```python
from build123d import *

# Parameters (mm, degrees)
SKETCH1_R                  = 31
BOSS_EXTRUDE1_DEPTH        = 4
F_3_2_3_2_DIAMETER_HOLE1_D = 3.2
F_3_0_3_DIAMETER_HOLE1_D   = 3
SKETCH6_W                  = 4
SKETCH6_H                  = 4
CUT_EXTRUDE2_DEPTH         = 45.022721406


with BuildPart() as part:
    # Sketch1 → Boss-Extrude1 (new body)
    with BuildSketch(Plane(origin=(0, 0, 0), x_dir=(1, 0, 0), z_dir=(0, 1, 0))):
        with Locations(Location((0, 0, 0), (0, 0, 270))):
            Circle(SKETCH1_R)
    extrude(amount=BOSS_EXTRUDE1_DEPTH)

    # Ø3.2 (3.2) Diameter Hole1 (through all)
    with Locations(Plane(origin=(0, 4, 0), x_dir=(1, 0, 0), z_dir=(0, 1, 0))):
        with Locations((-27.5, 0), (27.5, 0), (0, 27.5), (0, -27.5)):
            Hole(F_3_2_3_2_DIAMETER_HOLE1_D / 2)

    # Ø3.0 (3) Diameter Hole1 (through all)
    with Locations(Plane(origin=(0, 4, 0), x_dir=(1, 0, 0), z_dir=(0, 1, 0))):
        with Locations((-16.135, 0)):
            Hole(F_3_0_3_DIAMETER_HOLE1_D / 2)

    # Sketch6 → Cut-Extrude2 (cut, through all)
    with BuildSketch(Plane(origin=(0, 4, 0), x_dir=(1, 0, 0), z_dir=(0, 1, 0))):
        with Locations((0, 16.135)):
            Rectangle(SKETCH6_W, SKETCH6_H)
    extrude(amount=-CUT_EXTRUDE2_DEPTH, mode=Mode.SUBTRACT)


solid = part.part
```
Geometry: final body of the model. Coordinates: model frame, mm. A direction names the side the tool comes from. Coordinates: 2 decimals unless noted, no trailing zeros. Loops run counter-clockwise (first coordinate to the right, second up) from the corner with the lowest first, then second, coordinate; pieces in that order, holes last. Notation, with made-up numbers: M -21,41.25 L 5,41.25 A23 cw 5,64.25 Z; hole C -19.5,30 d2. An arc over 180 degrees is marked long. Put each result on its own line as item: value.
(1) Draft query along X for faces 1 (the face through (0, 4, 0)), 2 (the face through (30.736, 1.972, -4.036)), 3 (the face through (0, 2, -14.135)). Return one class per face: pulls with the +X half, pulls with the -X half, needs draft (parallel to the pull), parting line crosses it, or undercut.
Answer sheet:
face 1: needs draft
face 2: parting line crosses it
face 3: undercut
(2) First-contact query: pin 1 (2 mm diameter, centred on y = 2, z = -15.5, fed in from +X); pin 2 (1.5 mm diameter, centred on x = -10, y = 2, fed in from -Z); pin 3 (2 mm diameter, centred on x = -16, y = 2.5, fed in from -Z). Flat tips, straight axial feed; report the tip coordinate or a pass-through.
Answer sheet:
pin 1: stops at x = 27.4
pin 2: stops at z = -29.59
pin 3: stops at z = -27.13
(3) Access query for faces 4 (the face through (2, 2, -16)), 5 (the face through (0, 0, 0)). Directions: +Z, -Z, +X, -X, +Y, -Y. A direction counts if a zero-diameter tool reaches every point of the face in a straight line with its end or side. Return the directions, or none.
Answer sheet:
face 4: +Y, -Y
face 5: +Z, -Z, +X, -X, -Y
(4) Cut plane A-A on x = 0. Return the cut outline in (y, z) (3 decimals), then the cut area to 3 significant figures.
Answer sheet:
outline: M 0,-31 L 4,-31 L 4,-29.1 L 0,-29.1 Z; M 0,-25.9 L 4,-25.9 L 4,-18.135 L 0,-18.135 Z; M 0,-14.135 L 4,-14.135 L 4,25.9 L 0,25.9 Z; M 0,29.1 L 4,29.1 L 4,31 L 0,31 Z
area: 206 mm^2
(5) Cut plane B-B on z = 0. Return the cut outline in (x, y) (3 decimals), then the cut area to 3 significant figures.
Answer sheet:
outline: M -31,0 L -29.1,0 L -29.1,4 L -31,4 Z; M -25.9,0 L -17.635,0 L -17.635,4 L -25.9,4 Z; M -14.635,0 L 25.9,0 L 25.9,4 L -14.635,4 Z; M 29.1,0 L 31,0 L 31,4 L 29.1,4 Z
area: 210 mm^2
(6) Material intervals for probe 1 along X at (y, z) = (1.2, 27.5); probe 2 along Z at (x, y) = (-28, 2.35), sorted ascending.
Answer sheet:
probe 1: x = -14.31 to -1.6, 1.6 to 14.31
probe 2: z = -13.3 to -1.52, 1.52 to 13.3
(7) Cut plane D-D on x = -27.5. Return the cut outline in (y, z).
Answer sheet:
outline: M 0,-14.31 L 4,-14.31 L 4,-1.6 L 0,-1.6 Z; M 0,1.6 L 4,1.6 L 4,14.31 L 0,14.31 Z
(8) Cut plane C-C on y = 3.15. Return the cut outline in (x, z) (3 decimals), then the cut area to 3 significant figures.
Answer sheet:
outline: C 0,0 d62; hole C -27.5,0 d3.2; hole C -16.135,0 d3; hole M -2,-18.135 L 2,-18.135 L 2,-14.135 L -2,-14.135 Z; hole C 0,-27.5 d3.2; hole C 0,27.5 d3.2; hole C 27.5,0 d3.2
area: 2,960 mm^2
